Autodesk Inventor part; units mm, degrees
ref_plane "YZ Plane" through (0, 0, 0) normal (1, 0, 0) x (0, 1, 0)
ref_plane "XZ Plane" through (0, 0, 0) normal (0, 1, 0) x (-1, 0, 0)
ref_plane "XY Plane" through (0, 0, 0) normal (0, 0, 1) x (1, 0, 0)
sketch "草图1" plane through (0, 0, 0) normal (0, 0, 1) x (1, 0, 0)
  circle A0 centre (-1.9411, 0.0503) radius 2.5
  line L0 (4.3454, -10.9196) -> (9.6453, -10.9355)
  circle A1 centre (-1.9411, 0.0503) radius 5.5
  line L1 (-1.9411, -10.9276) -> (10.9921, -10.9276)
  line L2 (10.9921, -10.9276) -> (10.9921, 5.5503)
  line L3 (10.9921, 5.5503) -> (-1.9411, 5.5503)
  line L4 (-1.9411, 5.5503) -> (-1.9411, -10.9276)
  point P0 (6.9953, -10.9276)
  point P1 (-1.9411, 5.5503)
  point P2 (-1.9411, -5.4497)
  dimension "d3" = 3
  dimension "d5" = 5
extrude "拉伸1" add sketch "草图1" along normal blind 3.5 contours A0 L4 A1 | A0 L4 A1 | L3 L2 L1 L4 A1
fillet "圆角1" radius 4 1 edges at (-1.9411, -5.4497, 1.75)
sketch "草图2" plane through (0, 0, 0) normal (0, 0, -1) x (-1, 0, 0)
  point P0 (0, 0)
sketch "草图3" plane through (0, 0, 0) normal (0, 0, -1) x (-1, 0, 0)
  circle A0 centre (1.9411, 0.0503) radius 2.5
  circle A1 centre (1.9411, 0.0503) radius 4
  point P0 (0, 0)
  dimension "d6" = 8
extrude "拉伸2" cut sketch "草图3" against normal blind 1 contours A0 | A1
sketch "草图4" plane through (-1.9411, -10.9276, 0) normal (0, -1, 0) x (1, 0, 0)
  ellipse E0 centre (8.9346, 1.75) end of major axis (8.9346, 0.85) minor radius 0.9
  point P0 (1.9411, 0)
extrude "拉伸3" cut sketch "草图4" against normal blind 3
fillet "圆角2" radius 1 2 edges at (10.9921, 5.5503, 1.75) (-1.9411, -10.9276, 1.75)
sketch "草图5" plane through (0, 0, 3.5) normal (0, 0, 1) x (1, 0, 0)
  line L0 (15.1126, -4.4497) -> (15.1126, -8.4497)
  line L1 (5.3617, -4.4497) -> (15.1126, -4.4497)
  line L2 (5.3617, -8.4497) -> (5.3617, -4.4497)
  line L3 (5.3617, -8.4497) -> (15.1126, -8.4497)
  line L4 (5.3617, -6.4497) -> (10.3955, -6.4497)
  circle A0 centre (7.8786, -6.4497) radius 1
  circle A1 centre (7.8786, -6.4497) radius 1
  point P0 (0, 0)
  dimension "d12" = 2
extrude "拉伸4" cut sketch "草图5" against normal blind 5.5 contours A0 L4 | L4 A0
sketch "草图6" plane through (0, 0, 3.5) normal (0, 0, 1) x (1, 0, 0)
  circle A0 centre (7.8786, -2.4497) radius 1
  point P0 (0, 0)
extrude "拉伸5" cut sketch "草图6" against normal blind 10
properties part number "针头装配体"
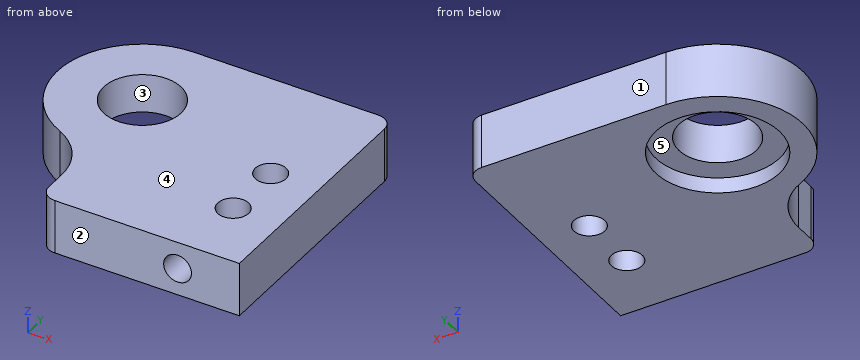
Geometry check sheet. Reference: the model listing, model coordinates, mm. Face numbers are marked on the shaded views. A direction names the side the tool comes from. Round coordinates to 2 decimals unless told otherwise and drop trailing zeros. Order: outer loops, then holes, each group sorted by start corner. A loop starts at its lowest first (then second) coordinate and runs counter-clockwise, first axis right, second up. Notation, with made-up numbers: (81.5, -34) - (106.5, -34) arc R16 ccw to (106.5, -26) - close; hole circle Ø9 at (86, 27). An arc over 180 degrees is marked (long way). One line per question, with ' | ' between items. Start each with the question number.
(1) Sectioned sample at C-C on x = -4.75. Record the cut outline in (y, z).
(2) Depth check by flat-ended pin: pin 1 Ø1.8 at (x, y) = (7.88, -6.45) entering from +Z; pin 2 Ø2 at (y, z) = (-3, 0.5) entering from -X; pin 3 Ø0.9 at (x, z) = (7, 2) entering from -Y; pin 4 Ø6.5 at (x, y) = (-1.94, 0.05) entering from -Z. Enter the tip coordinate at first touch or a pass-through.
(3) Release check for a two-part mould opening along Y. For the marked faces 1, 2 and 3 record: released by +Y, released by -Y, zero draft, split by the parting line, or undercut.
(4) Thickness scan on L1, parallel to Y at x = 8, z = 3.3; L2, parallel to X at y = -2, z = 0.95; L3, parallel to X at y = -6.5, z = 2.55. Record the ranges inside material, lowest first. Write a range as [from, to].
(5) Sectioned sample at B-B on z = 3.25. Record the cut outline in (x, y), and give its area (3 significant figures).
(6) Sectioned sample at D-D on y = 0.5. Record the cut outline in (x, z).
(7) Sectioned sample at A-A on y = 2.25. Record the cut outline in (x, z).
(8) Access from +Z, -Z, +X, -X, +Y, -Y to the whole of each face (thin tool, end or side, straight path). Record for the marked faces 4 and 5.
Conclusion:
1) outline: (-4.68, 0) - (-2.8, 0) - (-2.8, 1) - (2.9, 1) - (2.9, 0) - (4.78, 0) - (4.78, 3.5) - (-4.68, 3.5) - close
2) pin 1: passes through | pin 2: stops at x = -7.04 | pin 3: stops at y = -7.93 | pin 4: stops at z = 1
3) face 1: released by +Y | face 2: released by -Y | face 3: undercut
4) L1: y = [-10.93, -7.44], [-5.46, -3.44], [-1.46, 5.55] | L2: x = [-7.04, -5.38], [1.49, 6.99], [8.77, 10.99] | L3: x = [-2.52, 6.88], [8.88, 10.99]
5) outline: (-4.26, -4.94) arc R4 cw to (-1.94, -8.57) - (-1.94, -9.93) arc R1 ccw to (-0.94, -10.93) - (10.99, -10.93) - (10.99, 4.55) arc R1 ccw to (9.99, 5.55) - (-1.94, 5.55) arc R5.5 ccw to start; hole circle Ø5 at (-1.94, 0.05); hole circle Ø2 at (7.88, -6.45); hole circle Ø2 at (7.88, -2.45) | area: 236 mm2
6) outline: (-7.42, 0) - (-5.92, 0) - (-5.92, 1) - (-4.4, 1) - (-4.4, 3.5) - (-7.42, 3.5) - close; (0.52, 1) - (2.03, 1) - (2.03, 0) - (10.99, 0) - (10.99, 3.5) - (0.52, 3.5) - close
7) outline: (-6.98, 0) - (-5.28, 0) - (-5.28, 1) - (-3.13, 1) - (-3.13, 3.5) - (-6.98, 3.5) - close; (-0.75, 1) - (1.4, 1) - (1.4, 0) - (10.99, 0) - (10.99, 3.5) - (-0.75, 3.5) - close
8) face 4: +Z, +X, -X, +Y, -Y | face 5: -Z
